Part model, mm, in its own coordinate system. Coordinates: 2 decimals unless noted, no trailing zeros. Order: outer loops, then holes, each group sorted by start corner. A loop starts at its lowest first (then second) coordinate and runs counter-clockwise, first axis right, second up.
from build123d import *

# Parameters (mm, degrees)
SKETCH2_W           = 250
SKETCH2_H           = 286.5
BOSS_EXTRUDE1_DEPTH = 5
SKETCH3_R           = 2.5
SKETCH3_W           = 70
SKETCH3_H           = 25
CUT_EXTRUDE1_DEPTH  = 5


with BuildPart() as part:
    # Sketch2 → Boss-Extrude1 (new body)
    with BuildSketch(Plane.XY):
        Rectangle(SKETCH2_W, SKETCH2_H)
    extrude(amount=BOSS_EXTRUDE1_DEPTH)

    # Sketch3 → Cut-Extrude1 (cut)
    with BuildSketch(Plane.XY.offset(5)):
        with Locations((-110, -132.85)):
            Circle(SKETCH3_R)
        with Locations((-110, -107.85)):
            Circle(SKETCH3_R)
        with Locations((-110, 132.85)):
            Circle(SKETCH3_R)
        with Locations((-110, 107.85)):
            Circle(SKETCH3_R)
        with Locations((45, -130.75)):
            Rectangle(SKETCH3_W, SKETCH3_H)
        with Locations((45, 130.75)):
            Rectangle(SKETCH3_W, SKETCH3_H)
        with BuildLine():
            Line((28.31193033, 58.769897179), (12.096931793, 33.25))
            Line((12.096931793, 33.25), (47.903068207, 33.25))
            Line((47.903068207, 33.25), (31.68806967, 58.769897179))
            ThreePointArc((31.68806967, 58.769897179), (30, 59.697320474), (28.31193033, 58.769897179))
        make_face()
        with BuildLine():
            Line((23.394573112, 71.822576705), (5, 100.772786809))
            Line((5, 100.772786809), (5, 40.727213191))
            Line((5, 40.727213191), (23.394573112, 69.677423295))
            ThreePointArc((23.394573112, 69.677423295), (23.706503442, 70.75), (23.394573112, 71.822576705))
        make_face()
        with BuildLine():
            Line((47.903068207, 108.25), (12.096931793, 108.25))
            Line((12.096931793, 108.25), (28.31193033, 82.730102821))
            ThreePointArc((28.31193033, 82.730102821), (30, 81.802679526), (31.68806967, 82.730102821))
            Line((31.68806967, 82.730102821), (47.903068207, 108.25))
        make_face()
        with BuildLine():
            Line((-12.096931793, 108.25), (-47.903068207, 108.25))
            Line((-47.903068207, 108.25), (-31.68806967, 82.730102821))
            ThreePointArc((-31.68806967, 82.730102821), (-30, 81.802679526), (-28.31193033, 82.730102821))
            Line((-28.31193033, 82.730102821), (-12.096931793, 108.25))
        make_face()
        with BuildLine():
            Line((-5, 40.727213191), (-5, 100.772786809))
            Line((-5, 100.772786809), (-23.394573112, 71.822576705))
            ThreePointArc((-23.394573112, 71.822576705), (-23.706503442, 70.75), (-23.394573112, 69.677423295))
            Line((-23.394573112, 69.677423295), (-5, 40.727213191))
        make_face()
        with BuildLine():
            Line((-36.605426888, 71.822576705), (-55, 100.772786809))
            Line((-55, 100.772786809), (-55, 40.727213191))
            Line((-55, 40.727213191), (-36.605426888, 69.677423295))
            ThreePointArc((-36.605426888, 69.677423295), (-36.293496558, 70.75), (-36.605426888, 71.822576705))
        make_face()
        with BuildLine():
            Line((-31.68806967, 58.769897179), (-47.903068207, 33.25))
            Line((-47.903068207, 33.25), (-12.096931793, 33.25))
            Line((-12.096931793, 33.25), (-28.31193033, 58.769897179))
            ThreePointArc((-28.31193033, 58.769897179), (-30, 59.697320474), (-31.68806967, 58.769897179))
        make_face()
        with BuildLine():
            Line((55, 40.727213191), (55, 100.772786809))
            Line((55, 100.772786809), (36.605426888, 71.822576705))
            ThreePointArc((36.605426888, 71.822576705), (36.293496558, 70.75), (36.605426888, 69.677423295))
            Line((36.605426888, 69.677423295), (55, 40.727213191))
        make_face()
        with BuildLine():
            Line((-12.096931793, -33.25), (-47.903068207, -33.25))
            Line((-47.903068207, -33.25), (-31.68806967, -58.769897179))
            ThreePointArc((-31.68806967, -58.769897179), (-30, -59.697320474), (-28.31193033, -58.769897179))
            Line((-28.31193033, -58.769897179), (-12.096931793, -33.25))
        make_face()
        with BuildLine():
            Line((-36.605426888, -69.677423295), (-55, -40.727213191))
            Line((-55, -40.727213191), (-55, -100.772786809))
            Line((-55, -100.772786809), (-36.605426888, -71.822576705))
            ThreePointArc((-36.605426888, -71.822576705), (-36.293496558, -70.75), (-36.605426888, -69.677423295))
        make_face()
        with BuildLine():
            Line((-31.68806967, -82.730102821), (-47.903068207, -108.25))
            Line((-47.903068207, -108.25), (-12.096931793, -108.25))
            Line((-12.096931793, -108.25), (-28.31193033, -82.730102821))
            ThreePointArc((-28.31193033, -82.730102821), (-30, -81.802679526), (-31.68806967, -82.730102821))
        make_face()
        with BuildLine():
            Line((-5, -100.772786809), (-5, -40.727213191))
            Line((-5, -40.727213191), (-23.394573112, -69.677423295))
            ThreePointArc((-23.394573112, -69.677423295), (-23.706503442, -70.75), (-23.394573112, -71.822576705))
            Line((-23.394573112, -71.822576705), (-5, -100.772786809))
        make_face()
        with BuildLine():
            Line((23.394573112, -69.677423295), (5, -40.727213191))
            Line((5, -40.727213191), (5, -100.772786809))
            Line((5, -100.772786809), (23.394573112, -71.822576705))
            ThreePointArc((23.394573112, -71.822576705), (23.706503442, -70.75), (23.394573112, -69.677423295))
        make_face()
        with BuildLine():
            Line((47.903068207, -33.25), (12.096931793, -33.25))
            Line((12.096931793, -33.25), (28.31193033, -58.769897179))
            ThreePointArc((28.31193033, -58.769897179), (30, -59.697320474), (31.68806967, -58.769897179))
            Line((31.68806967, -58.769897179), (47.903068207, -33.25))
        make_face()
        with BuildLine():
            Line((55, -100.772786809), (55, -40.727213191))
            Line((55, -40.727213191), (36.605426888, -69.677423295))
            ThreePointArc((36.605426888, -69.677423295), (36.293496558, -70.75), (36.605426888, -71.822576705))
            Line((36.605426888, -71.822576705), (55, -100.772786809))
        make_face()
        with BuildLine():
            Line((28.31193033, -82.730102821), (12.096931793, -108.25))
            Line((12.096931793, -108.25), (47.903068207, -108.25))
            Line((47.903068207, -108.25), (31.68806967, -82.730102821))
            ThreePointArc((31.68806967, -82.730102821), (30, -81.802679526), (28.31193033, -82.730102821))
        make_face()
        with BuildLine():
            Line((83.394573112, -69.677423295), (65, -40.727213191))
            Line((65, -40.727213191), (65, -100.772786809))
            Line((65, -100.772786809), (83.394573112, -71.822576705))
            ThreePointArc((83.394573112, -71.822576705), (83.706503442, -70.75), (83.394573112, -69.677423295))
        make_face()
        with BuildLine():
            Line((107.903068207, -33.25), (72.096931793, -33.25))
            Line((72.096931793, -33.25), (88.31193033, -58.769897179))
            ThreePointArc((88.31193033, -58.769897179), (90, -59.697320474), (91.68806967, -58.769897179))
            Line((91.68806967, -58.769897179), (107.903068207, -33.25))
        make_face()
        with BuildLine():
            Line((115, -100.772786809), (115, -40.727213191))
            Line((115, -40.727213191), (96.605426888, -69.677423295))
            ThreePointArc((96.605426888, -69.677423295), (96.293496558, -70.75), (96.605426888, -71.822576705))
            Line((96.605426888, -71.822576705), (115, -100.772786809))
        make_face()
        with BuildLine():
            Line((88.31193033, -82.730102821), (72.096931793, -108.25))
            Line((72.096931793, -108.25), (107.903068207, -108.25))
            Line((107.903068207, -108.25), (91.68806967, -82.730102821))
            ThreePointArc((91.68806967, -82.730102821), (90, -81.802679526), (88.31193033, -82.730102821))
        make_face()
        with BuildLine():
            Line((115, 40.727213191), (115, 100.772786809))
            Line((115, 100.772786809), (96.605426888, 71.822576705))
            ThreePointArc((96.605426888, 71.822576705), (96.293496558, 70.75), (96.605426888, 69.677423295))
            Line((96.605426888, 69.677423295), (115, 40.727213191))
        make_face()
        with BuildLine():
            Line((91.68806967, 82.730102821), (107.903068207, 108.25))
            Line((107.903068207, 108.25), (72.096931793, 108.25))
            Line((72.096931793, 108.25), (88.31193033, 82.730102821))
            ThreePointArc((88.31193033, 82.730102821), (90, 81.802679526), (91.68806967, 82.730102821))
        make_face()
        with BuildLine():
            Line((83.394573112, 71.822576705), (65, 100.772786809))
            Line((65, 100.772786809), (65, 40.727213191))
            Line((65, 40.727213191), (83.394573112, 69.677423295))
            ThreePointArc((83.394573112, 69.677423295), (83.706503442, 70.75), (83.394573112, 71.822576705))
        make_face()
        with BuildLine():
            Line((72.096931793, 33.25), (107.903068207, 33.25))
            Line((107.903068207, 33.25), (91.68806967, 58.769897179))
            ThreePointArc((91.68806967, 58.769897179), (90, 59.697320474), (88.31193033, 58.769897179))
            Line((88.31193033, 58.769897179), (72.096931793, 33.25))
        make_face()
    extrude(amount=-CUT_EXTRUDE1_DEPTH, mode=Mode.SUBTRACT)


solid = part.part
Q1. Pin check, flat tip, straight feed: pin 1 Ø1.5 at (x, z) = (42.5, 1.5) entering from -Y. Stop position of the tip, or through.
Results list:
pin 1: stops at y = -118.25
Q2. Cut at A-A on y = 121.5. Write the cut outline in (x, z), and give its area (3 significant figures).
Results list:
outline: (-125, 0) - (10, 0) - (10, 5) - (-125, 5) - close; (80, 0) - (125, 0) - (125, 5) - (80, 5) - close
area: 900 mm2
Q3. Cut at B-B on z = 1. Count the separate pieces of the cut face and the enclosed holes in it, and give its area (3 significant figures).
Results list:
separate pieces: 1
enclosed holes: 28
area: 55,200 mm2
Q4. Wall check: line 1 along X through (y, z) = (132.85, 2.95); line 2 along Y through (x, z) = (-110, 3.6); line 3 along Y through (x, z) = (112.5, 2.1). Give the ranges that are in metal, low to high.
Results list:
line 1: x = -125 to -112.5, -107.5 to 10, 80 to 125
line 2: y = -143.25 to -135.35, -130.35 to -110.35, -105.35 to 105.35, 110.35 to 130.35, 135.35 to 143.25
line 3: y = -143.25 to -96.84, -44.66 to 44.66, 96.84 to 143.25
